CAD build for the part. Positions are in the model's coordinates, mm. Give positions to 0.01 mm unless a question says otherwise; leave off trailing zeros. Write each loop counter-clockwise with the first axis right and the second up, starting at its lowest first coordinate (ties: lowest second). Pieces come first, ordered by that corner, then holes. Notation, with made-up numbers: (-7, 4.25) - (9, 4.25) arc R7 ccw to (9, 13.25) - close; hole circle Ø8 at (83, 55.5). An arc over 180 degrees is marked (long way). Answer as a JSON object with one key per item and string values.
from build123d import *

# Parameters (mm, degrees)
F0_W     = 300
F0_H     = 180
F0_R     = 10
F1_DEPTH = 25
F2_SIZE2 = 2
F2_SIZE  = 2
F3_SIZE2 = 2
F3_SIZE  = 2


with BuildPart() as f1:
    # F0 (on Front) → F1 (new body)
    with BuildSketch(Plane.XZ):
        with Locations((150, 90)):
            Rectangle(F0_W, F0_H)
        with Locations((25, 25)):
            Circle(F0_R, mode=Mode.SUBTRACT)
        with Locations((150, 25)):
            Circle(F0_R, mode=Mode.SUBTRACT)
        with Locations((275, 25)):
            Circle(F0_R, mode=Mode.SUBTRACT)
        with Locations((25, 155)):
            Circle(F0_R, mode=Mode.SUBTRACT)
        with Locations((150, 155)):
            Circle(F0_R, mode=Mode.SUBTRACT)
        with Locations((275, 155)):
            Circle(F0_R, mode=Mode.SUBTRACT)
    extrude(amount=F1_DEPTH)

    # F2
    f2_edges = [f1.edges().sort_by_distance(p)[0] for p in [
        (15, -25, 155),
        (15, -25, 25),
        (140, -25, 25),
        (140, -25, 155),
        (265, -25, 155),
        (265, -25, 25),
    ]]
    chamfer(f2_edges, length=F2_SIZE, length2=F2_SIZE2)

    # F3
    f3_edges = [f1.edges().sort_by_distance(p)[0] for p in [
        (300, -25, 90),
        (150, -25, 0),
        (0, -25, 90),
        (150, -25, 180),
        (150, 0, 0),
        (0, 0, 90),
        (300, 0, 90),
        (150, 0, 180),
    ]]
    chamfer(f3_edges, length=F3_SIZE, length2=F3_SIZE2)


solid = f1.part
(1) Saw through at B-B, the plane y = -18.25. Give the cut face in (x, z).
Answer key:
{"outline": "(0, 0) - (300, 0) - (300, 180) - (0, 180) - close; hole circle Ø20 at (25, 25); hole circle Ø20 at (25, 155); hole circle Ø20 at (150, 25); hole circle Ø20 at (150, 155); hole circle Ø20 at (275, 25); hole circle Ø20 at (275, 155)"}
(2) Saw through at A-A, the plane x = 25. Give the cut face in (y, z), and give its area (3 significant figures).
Answer key:
{"outline": "(-25, 2) - (-23, 0) - (-2, 0) - (0, 2) - (0, 15) - (-23, 15) - (-25, 13) - close; (-25, 37) - (-23, 35) - (0, 35) - (0, 145) - (-23, 145) - (-25, 143) - close; (-25, 167) - (-23, 165) - (0, 165) - (0, 178) - (-2, 180) - (-23, 180) - (-25, 178) - close", "area": "3,480 mm²"}
(3) Saw through at C-C, the plane z = 155. Give the cut face in (x, y).
Answer key:
{"outline": "(0, -23) - (2, -25) - (13, -25) - (15, -23) - (15, 0) - (2, 0) - (0, -2) - close; (35, -23) - (37, -25) - (138, -25) - (140, -23) - (140, 0) - (35, 0) - close; (160, -23) - (162, -25) - (263, -25) - (265, -23) - (265, 0) - (160, 0) - close; (285, -23) - (287, -25) - (298, -25) - (300, -23) - (300, -2) - (298, 0) - (285, 0) - close"}
(4) Probe L1, parallel to Z at x = 275, y = -7.75; L2, parallel to X at y = -2.5, z = 22.5. List the from-to ranges inside material, lowest first. Write a range as [from, to].
Answer key:
{"L1": "z = [0, 15], [35, 145], [165, 180]", "L2": "x = [0, 15.32], [34.68, 140.32], [159.68, 265.32], [284.68, 300]"}
(5) Pull direction Z, two halves, no side cores. Call faces 1 (the face through (17.537, -23.125, 161.843)), 2 (the face through (148, -12, 0)), 3 (the face through (284.54, -11.34, 28)), 4 (the face through (148, 0, 91)): pulls with the +Z half, pulls with the -Z half, needs draft (parallel to the pull), parting line crosses it, or undercut.
Answer key:
{"face 1": "undercut", "face 2": "pulls with the -Z half", "face 3": "undercut", "face 4": "needs draft"}
(6) Flat gauge pin, fed straight in: P1, Ø12, axis at x = 25, z = 25, coming from the +Y side. Where does the tip first touch, or does it go through?
Answer key:
{"P1": "passes through"}
